```python
from build123d import *

# Parameters (mm, degrees)
SKETCH1_W                = 107.95
SKETCH1_H                = 220.345
EXTRUDE1_DEPTH           = 31.75
EXTRUDE2_DEPTH           = 20.955
EXTRUDE2_DEPTH_BACK      = 52.705
SKETCH2_R                = 58.674
SKETCH3_R                = 36.5125
EXTRUDE3_DEPTH           = 223.438643032
F_5_16_24_TAPPED_HOLE1_D = 6.9088
CIRPATTERN1_COUNT        = 10
EXTRUDE4_DEPTH           = 20.955
EXTRUDE4_DEPTH_BACK      = 20.955
SKETCH7_W                = 132.842
SKETCH7_H                = 55.172869126
SKETCH8_R                = 23.174591889
EXTRUDE5_DEPTH           = 114.3


with BuildPart() as part:
    # Sketch1 → Extrude1 (new body)
    with BuildSketch(Plane.XY):
        with Locations((24.778661236, -82.412046749)):
            Rectangle(SKETCH1_W, SKETCH1_H)
    extrude(amount=EXTRUDE1_DEPTH)

    # Sketch2 → Extrude2 (add, two sides: drawn at the far end of the back side and taken through both)
    with BuildSketch(Plane.XY.offset(31.75).offset(-EXTRUDE2_DEPTH_BACK)):
        with Locations((24.778661236, -127.052546749)):
            Circle(SKETCH2_R)
    extrude(amount=EXTRUDE2_DEPTH + EXTRUDE2_DEPTH_BACK)

    # Sketch3 → Extrude3 (cut, through all)
    with BuildSketch(Plane.XY.offset(52.705)):
        with Locations((24.778661236, -127.052546749)):
            Circle(SKETCH3_R)
    extrude(amount=-EXTRUDE3_DEPTH, mode=Mode.SUBTRACT)

    # 5/16-24 Tapped Hole1 (through all)
    with Locations(Plane.XY.offset(52.705)):
        with Locations((8.962862447, -78.376523189)):
            f_5_16_24_tapped_hole1 = Hole(F_5_16_24_TAPPED_HOLE1_D / 2)

    # CirPattern1: 5/16-24 Tapped Hole1 ×10 about axis
    cirpattern1_axis = Axis((24.778661236, -127.052546749, 0), (0, 0, 1))
    for i in range(1, CIRPATTERN1_COUNT):
        add(f_5_16_24_tapped_hole1.rotate(cirpattern1_axis, i * 360 / CIRPATTERN1_COUNT), mode=Mode.SUBTRACT)

    # Sketch7 → Extrude4 (add, two sides: drawn at the far end of the back side and taken through both)
    with BuildSketch(Plane(origin=(0, 27.760453251, 0), x_dir=(1, 0, 0), z_dir=(0, 1, 0)).offset(-EXTRUDE4_DEPTH_BACK)):
        with Locations((24.778661236, -15.875)):
            Rectangle(SKETCH7_W, SKETCH7_H)
    extrude(amount=EXTRUDE4_DEPTH + EXTRUDE4_DEPTH_BACK)

    # Sketch8 → Extrude5 (add)
    with BuildSketch(Plane(origin=(0, 48.715453251, 0), x_dir=(1, 0, 0), z_dir=(0, 1, 0))):
        with Locations(Location((55.144248721, -16.946726617, 0), (0, 0, 90))):
            Circle(SKETCH8_R)
    extrude(amount=EXTRUDE5_DEPTH)


solid = part.part
```
Input: part model. Units: mm. Frame: model coordinates. A direction names the side the tool comes from. Give positions to 0.01 mm unless a question says otherwise; leave off trailing zeros. Order: outer loops, then holes, each group sorted by start corner. A loop starts at its lowest first (then second) coordinate and runs counter-clockwise, first axis right, second up. Notation, with made-up numbers: M -35,88 L 3,88 A20 ccw 3,99 Z; hole C 84,6.5 d11. An arc over 180 degrees is marked long. Return JSON: item names as keys, results as strings.
1) Contact query for flat-ended pins moving along their axis: pin 1 (4 mm diameter, centred on x = -16.63, y = -157.14, fed in from +Z); pin 2 (8 mm diameter, centred on x = -5, y = -27, fed in from -Z); pin 3 (9.5 mm diameter, centred on y = -29.5, z = 15.5, fed in from +X); pin 4 (5 mm diameter, centred on x = 72.5, y = -76.5, fed in from +Z). Output: stop coordinate, or through.
Taken from the geometry:
{"pin 1": "passes through", "pin 2": "stops at z = 0", "pin 3": "stops at x = 78.75", "pin 4": "stops at z = 31.75"}
2) Section query A-A on y = -137.5. Output: boundary loops of the cut face in (x, z) (3 decimals).
Taken from the geometry:
{"outline": "M -32.958,-20.955 L -10.207,-20.955 L -10.207,52.705 L -32.958,52.705 Z; M 59.765,-20.955 L 82.515,-20.955 L 82.515,52.705 L 59.765,52.705 Z"}
3) Access query for faces 1 (the face through (24, -190, 31.75)), 2 (the face through (24, -190, 0)), 3 (the face through (24, 27, -11.711)), 4 (the face through (78.754, -49, 16)). Directions: +Z, -Z, +X, -X, +Y, -Y. A direction counts if a zero-diameter tool reaches every point of the face in a straight line with its end or side. Return the directions, or none.
Taken from the geometry:
{"face 1": "+Z, -Y", "face 2": "-Z, -Y", "face 3": "-Z, +X, -X, +Y", "face 4": "+Z, -Z, +X"}
4) Line query: L1, parallel to Y at x = 15, z = -11.5; L2, parallel to Y at x = -17.5, z = 48; L3, parallel to Z at x = -9, y = 18. Output: solid intervals per line, ascending. Write a range as [from, to].
Taken from the geometry:
{"L1": "y = [-184.91, -162.23], [-91.87, -69.2], [6.81, 48.72]", "L2": "y = [-167.74, -160.48], [-153.79, -100.31], [-93.63, -86.37]", "L3": "z = [-11.71, 43.46]"}
5) Mould query, pull axis Y, two halves, no side actions, for faces 5 (the face through (-29.196, -172, 16)), 6 (the face through (40.145, -179.154, 15.359)), 7 (the face through (24, -192.585, 16)). Classes: released by +Y, released by -Y, zero draft, split by the parting line, or undercut.
Taken from the geometry:
{"face 5": "zero draft", "face 6": "undercut", "face 7": "released by -Y"}
6) Section query C-C on z = 28. Count the separate pieces of the cut face and the enclosed holes in it, and give its area (3 significant figures).
Taken from the geometry:
{"separate pieces": "1", "enclosed holes": "11", "area": "27,500 mm2"}
7) Section query D-D on y = -6. Output: boundary loops of the cut face in (x, z).
Taken from the geometry:
{"outline": "M -29.2,0 L 78.75,0 L 78.75,31.75 L -29.2,31.75 Z"}
